Drawing for the job (mm, zero at the part's lowest x, y, z). A direction names the side the tool comes from. Round coordinates to 2 decimals unless told otherwise and drop trailing zeros. Order: outer loops, then holes, each group sorted by start corner. A loop starts at its lowest first (then second) coordinate and runs counter-clockwise, first axis right, second up. Notation, with made-up numbers: (-17, -6.5) - (-12, -6.5) arc R25 cw to (-12, 15.5) - close; hole circle Ø2 at (30.5, 26). An arc over 180 degrees is marked (long way). Put each result on its own line as item: value. Start each with the question number.
Item 1: Saw through at C-C on y = 17.5. List the corners of the cut face in (x, z).
Item 2: Pin check, flat tips, straight feed: pin 1 Ø0.9 at (x, z) = (3.5, 33.5) entering from -Y; pin 2 Ø12.5 at (x, z) = (9.5, 20.5) entering from -Y. Stop position of each tip, or through.
Item 3: Which spindle directions (+Z, -Z, +X, -X, +Y, -Y) get a long thin tool onto all of the face, cutting with end or side? Do the marked faces 1 and 2. Say none if no direction does.
Item 4: Mould opens along Z. For the marked faces 3, 4, 5 and 6 say: pulls with the +Z half, pulls with the -Z half, needs draft (parallel to the pull), parting line crosses it, or undercut.
Item 5: Probe probe 1 along Z at (x, y) = (16, 21.5); probe 2 along Y at (x, z) = (32, 23); probe 3 along Y at (x, z) = (18, 34). List the from-to ranges inside material, lowest first.
Item 6: Saw through at B-B on z = 17.5. List the corners of the cut face in (x, y) (1 decimal).
Item 7: Saw through at D-D on x = 18.5. List the corners of the cut face in (y, z) (1 decimal).
Item 8: Saw through at A-A on y = 3.5. List the corners of the cut face in (x, z), plus the area to 3 significant figures.
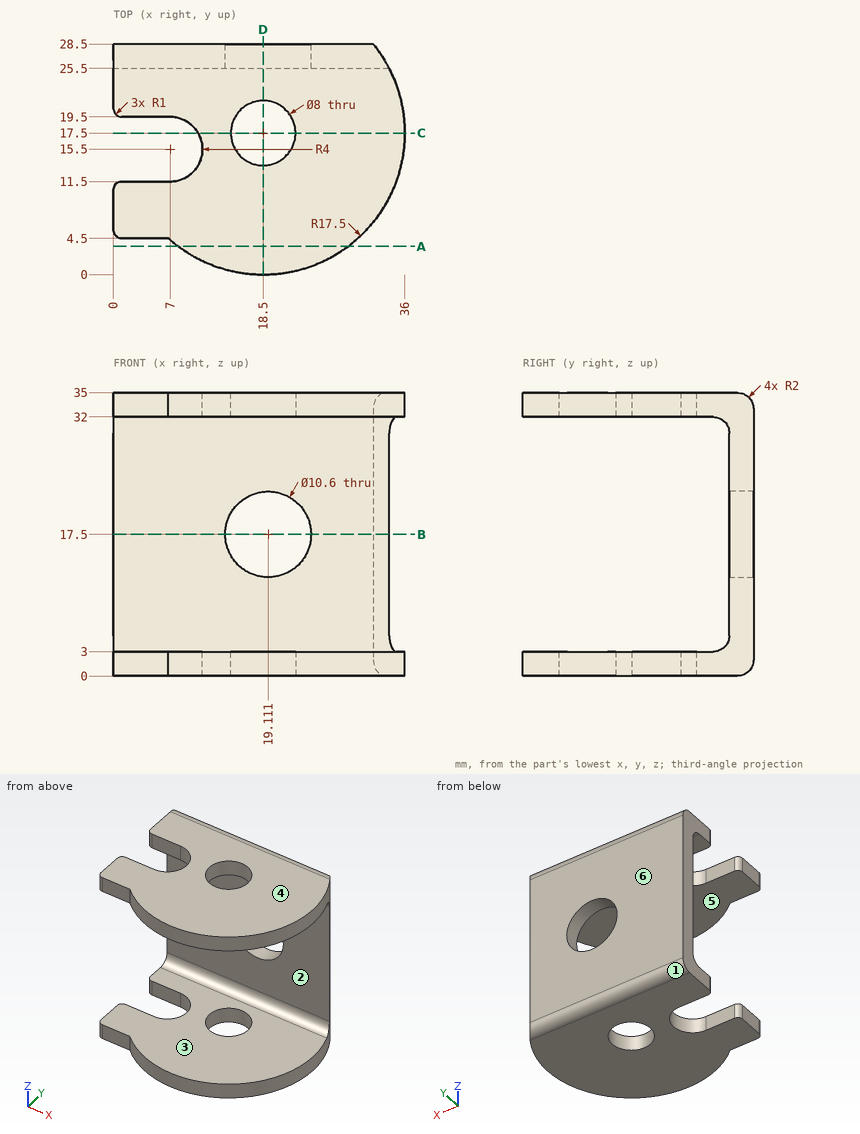
Results found:
1. outline: (10.46, 0) - (14.5, 0) - (14.5, 3) - (10.46, 3) - close; (10.46, 32) - (14.5, 32) - (14.5, 35) - (10.46, 35) - close; (22.5, 0) - (36, 0) - (36, 3) - (22.5, 3) - close; (22.5, 32) - (36, 32) - (36, 35) - (22.5, 35) - close
2. pin 1: stops at y = 4.5
2. pin 2: stops at y = 25.5
3. face 1: -Z, +X, -X, +Y
3. face 2: +X, -X, -Y
4. face 3: undercut
4. face 4: pulls with the +Z half
4. face 5: undercut
4. face 6: needs draft
5. probe 1: z = 0 to 3, 32 to 35
5. probe 2: y = 25.5 to 28.5
5. probe 3: y = 0.01 to 13.53, 21.47 to 28.23
6. outline: (0, 25.5) - (13.8, 25.5) - (13.8, 28.5) - (0, 28.5) - close; (24.4, 25.5) - (34.1, 25.5) arc R17.5 ccw to (32.1, 28.5) - (24.4, 28.5) - close
7. outline: (0, 0) - (13.5, 0) - (13.5, 3) - (0, 3) - close; (0, 32) - (13.5, 32) - (13.5, 35) - (0, 35) - close; (21.5, 0) - (26.5, 0) arc R2 ccw to (28.5, 2) - (28.5, 12.2) - (25.5, 12.2) - (25.5, 5) arc R2 cw to (23.5, 3) - (21.5, 3) - close; (21.5, 32) - (23.5, 32) arc R2 cw to (25.5, 30) - (25.5, 22.8) - (28.5, 22.8) - (28.5, 33) arc R2 ccw to (26.5, 35) - (21.5, 35) - close
8. outline: (8, 0) - (29, 0) - (29, 3) - (8, 3) - close; (8, 32) - (29, 32) - (29, 35) - (8, 35) - close
8. area: 126 mm²
